Could you check a few things on this model? Use its own coordinates, in mm. A direction names the side the tool comes from. Give positions to 0.01 mm unless a question says otherwise; leave off trailing zeros. Write each loop counter-clockwise with the first axis right and the second up, starting at its lowest first coordinate (ties: lowest second). Pieces come first, ordered by that corner, then holes. Notation, with made-up numbers: M 13.5,23.5 L 25.5,23.5 A19 ccw 25.5,50.5 Z; hole C -39,-12.75 d9. An arc over 180 degrees is marked long. Answer as a JSON object with one key per item and string values. Group by question number.
```python
from build123d import *

# Parameters (mm, degrees)
F0_W     = 26.67
F0_H     = 26.67
F1_DEPTH = 1.5875
F2_W     = 5.08
F2_H     = 5.08
F3_DEPTH = 1.651


with BuildPart() as f1:
    # F0 (on Right) → F1 (new body)
    with BuildSketch(Plane.YZ):
        with Locations((13.335, 13.335)):
            Rectangle(F0_W, F0_H)
    extrude(amount=F1_DEPTH)

    # F2 (on face) → F3 (join)
    with BuildSketch(Plane.YZ.offset(1.5875)):
        with Locations((4.572, 22.098)):
            Rectangle(F2_W, F2_H)
        with Locations((4.572, 13.2842)):
            Rectangle(F2_W, F2_H)
        with Locations((4.572, 4.4704)):
            Rectangle(F2_W, F2_H)
        with Locations((13.3858, 22.098)):
            Rectangle(F2_W, F2_H)
        with Locations((13.3858, 13.2842)):
            Rectangle(F2_W, F2_H)
        with Locations((13.3858, 4.4704)):
            Rectangle(F2_W, F2_H)
        with Locations((22.1996, 22.098)):
            Rectangle(F2_W, F2_H)
        with Locations((22.1996, 13.2842)):
            Rectangle(F2_W, F2_H)
        with Locations((22.1996, 4.4704)):
            Rectangle(F2_W, F2_H)
    extrude(amount=F3_DEPTH)


solid = f1.part
```
1) If we section it at D-D, the plane y = 9: List the corners of the cut face in (x, z) for me, plus the area to 3 significant figures.
2) For faces 4 (the flat face through (2, 13, 15.824)), 5 (the flat face through (2, 5, 1.93)), 6 (the flat face through (2, 10.846, 4)), 7 (the flat face through (2, 2.032, 13)), 8 (the flat face through (2, 5, 24.638)), which set-ups out of +Z, -Z, +X, -X, +Y, -Y let a thin tool reach every point of the face, with its end or its side?
3) If we section it at A-A, the plane z = 4.25: List the corners of the cut face in (x, y) for me.
4) If we section it at C-C, the plane x = 1.9: Give the number of separate pieces and of enclosed holes in the cut face, plus the area to 3 significant figures.
5) If we section it at B-B, the plane y = 13.5: List the corners of the cut face in (x, z) for me.
6) Please list where these lines run through material, in increasing order: line 1 along Z through (x, y) = (2, 3); line 2 along Y through (x, z) = (2.85, 22); line 3 along X through (y, z) = (18.75, 20.5). Write a range as from..to.
7) We'd pull the mould along Y, two halves only. Please class faces 1 (the flat face through (2, 10.846, 13)), 2 (the flat face through (2, 2.032, 22)), 3 (the flat face through (2, 5, 19.558)): released by +Y, released by -Y, zero draft, split by the parting line, or undercut.
8) I'm going to push flat-ended pins straight in: pin 1 (1.3 mm diameter, centred on x = 2.5, z = 22, fed in from +Y); pin 2 (0.5 mm diameter, centred on x = 2, z = 13, fed in from -Y); pin 3 (0.8 mm diameter, centred on x = 2.5, y = 4.5, fed in from +Z). Where does each tip first touch, or does it pass through?
Taken from the geometry:
{
 "1": {"outline": "M 0,0 L 1.59,0 L 1.59,26.67 L 0,26.67 Z", "area": "42.3 mm²"},
 "2": {"face 4": "+X, +Y, -Y", "face 5": "-Z, +X, +Y, -Y", "face 6": "+Z, -Z, +X", "face 7": "+Z, -Z, +X, -Y", "face 8": "+Z, +X, +Y, -Y"},
 "3": {"outline": "M 0,0 L 1.59,0 L 1.59,2.03 L 3.24,2.03 L 3.24,7.11 L 1.59,7.11 L 1.59,10.85 L 3.24,10.85 L 3.24,15.93 L 1.59,15.93 L 1.59,19.66 L 3.24,19.66 L 3.24,24.74 L 1.59,24.74 L 1.59,26.67 L 0,26.67 Z"},
 "4": {"separate pieces": "9", "enclosed holes": "0", "area": "232 mm²"},
 "5": {"outline": "M 0,0 L 1.59,0 L 1.59,1.93 L 3.24,1.93 L 3.24,7.01 L 1.59,7.01 L 1.59,10.74 L 3.24,10.74 L 3.24,15.82 L 1.59,15.82 L 1.59,19.56 L 3.24,19.56 L 3.24,24.64 L 1.59,24.64 L 1.59,26.67 L 0,26.67 Z"},
 "6": {"line 1": "1.93..7.01, 10.74..15.82, 19.56..24.64", "line 2": "2.03..7.11, 10.85..15.93, 19.66..24.74", "line 3": "0..1.59"},
 "7": {"face 1": "undercut", "face 2": "released by -Y", "face 3": "zero draft"},
 "8": {"pin 1": "y = 24.74", "pin 2": "y = 2.03", "pin 3": "z = 24.64"}
}
